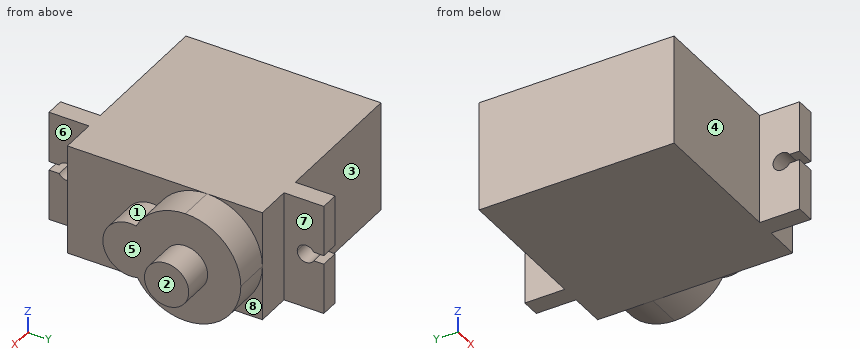
from build123d import *

# Parameters (mm, degrees)
F0_W      = 22
F0_H      = 22
F1_DEPTH  = 12.5
F3_DEPTH  = 4
F4_R      = 2.5
F5_DEPTH  = 3.5
F6_W      = 2.1
F6_H      = 12.5
F7_DEPTH  = 4.5
F9_DEPTH  = 2.1
F10_W     = 2.1
F10_H     = 12.5
F11_DEPTH = 4.5
F13_DEPTH = 2.1


with BuildPart() as f1:
    # F0 (on Top) → F1 (new body)
    with BuildSketch(Plane.XY):
        Rectangle(F0_W, F0_H)
    extrude(amount=F1_DEPTH)

    # F2 (on face) → F3 (join)
    with BuildSketch(Plane.YZ.offset(11)):
        with BuildLine():
            ThreePointArc((-0.6636140703, 3.1266552068), (1.6241725062, 0.8378190645), (4.75, 0))
            ThreePointArc((4.75, 0), (9.1694173824, 1.8305826176), (11, 6.25))
            ThreePointArc((11, 6.25), (9.1694173824, 10.6694173824), (4.75, 12.5))
            ThreePointArc((4.75, 12.5), (1.4810489541, 11.5769558905), (-0.8223385695, 9.0804668991))
            ThreePointArc((-0.8223385695, 9.0804668991), (0.9015416929, 8.0022024538), (1.5744178172, 6.0834385042))
            ThreePointArc((1.5744178172, 6.0834385042), (0.9518242766, 4.2292975847), (-0.6636140703, 3.1266552068))
        make_face()
        with BuildLine():
            ThreePointArc((-0.8223385695, 9.0804668991), (-4.568887039, 6.001564921), (-0.6636140703, 3.1266552068))
            ThreePointArc((-0.6636140703, 3.1266552068), (-1.4977801872, 6.0834385042), (-0.8223385695, 9.0804668991))
        make_face()
        with BuildLine():
            ThreePointArc((-0.8223385695, 9.0804668991), (-1.4977801872, 6.0834385042), (-0.6636140703, 3.1266552068))
            ThreePointArc((-0.6636140703, 3.1266552068), (0.9518242766, 4.2292975847), (1.5744178172, 6.0834385042))
            ThreePointArc((1.5744178172, 6.0834385042), (0.9015416929, 8.0022024538), (-0.8223385695, 9.0804668991))
        make_face()
    extrude(amount=F3_DEPTH)

    # F4 (on face) → F5 (join)
    with BuildSketch(Plane.YZ.offset(15)):
        with Locations((4.75, 6.25)):
            Circle(F4_R)
    extrude(amount=F5_DEPTH)

    # F6 (on face) → F7 (join)
    with BuildSketch(Plane.XZ.offset(11)):
        with Locations((5.95, 6.25)):
            Rectangle(F6_W, F6_H)
    extrude(amount=F7_DEPTH)

    # F8 (on face) → F9 (cut)
    with BuildSketch(Plane(origin=(4.9, 0, 0), x_dir=(0, -1, 0), z_dir=(-1, 0, 0))):
        with BuildLine():
            ThreePointArc((14.3660254038, 6.75), (14.4659258263, 6.5088190451), (14.5, 6.25))
            ThreePointArc((14.5, 6.25), (14.4659258263, 5.9911809549), (14.3660254038, 5.75))
            Line((14.3660254038, 5.75), (15.5, 5.75))
            Line((15.5, 5.75), (15.5, 6.75))
            Line((15.5, 6.75), (14.3660254038, 6.75))
        make_face()
        with BuildLine():
            ThreePointArc((14.3660254038, 5.75), (14.4659258263, 5.9911809549), (14.5, 6.25))
            ThreePointArc((14.5, 6.25), (14.4659258263, 6.5088190451), (14.3660254038, 6.75))
            ThreePointArc((14.3660254038, 6.75), (12.5, 6.25), (14.3660254038, 5.75))
        make_face()
    extrude(amount=-F9_DEPTH, mode=Mode.SUBTRACT)

    # F10 (on face) → F11 (join)
    with BuildSketch(Plane(origin=(0, 11, 0), x_dir=(-1, 0, 0), z_dir=(0, 1, 0))):
        with Locations((-5.95, 6.25)):
            Rectangle(F10_W, F10_H)
    extrude(amount=F11_DEPTH)

    # F12 (on face) → F13 (cut)
    with BuildSketch(Plane(origin=(4.9, 0, 0), x_dir=(0, -1, 0), z_dir=(-1, 0, 0))):
        with BuildLine():
            ThreePointArc((-14.3660254038, 5.75), (-13.2411809549, 5.2840741737), (-12.5, 6.25))
            ThreePointArc((-12.5, 6.25), (-13.2411809549, 7.2159258263), (-14.3660254038, 6.75))
            ThreePointArc((-14.3660254038, 6.75), (-14.5, 6.25), (-14.3660254038, 5.75))
        make_face()
        with BuildLine():
            ThreePointArc((-14.3660254038, 5.75), (-14.5, 6.25), (-14.3660254038, 6.75))
            Line((-14.3660254038, 6.75), (-15.5, 6.75))
            Line((-15.5, 6.75), (-15.5, 5.75))
            Line((-15.5, 5.75), (-14.3660254038, 5.75))
        make_face()
    extrude(amount=-F13_DEPTH, mode=Mode.SUBTRACT)


solid = f1.part
Design review of the part built by this model. Coordinates are the model's own, in mm. Face numbers are marked on the shaded views. A direction names the side the tool comes from. Round coordinates to 2 decimals unless told otherwise and drop trailing zeros. Loops run counter-clockwise (first coordinate to the right, second up) from the corner with the lowest first, then second, coordinate; pieces in that order, holes last. Notation, with made-up numbers: (13, 80) -> (52, 80) arc R28 ccw to (52, 99) -> close; hole circle Ø8 at (-3.5, -35). An arc over 180 degrees is marked (long way). Use one line per item in the form item = value. Start each with the question number.
Q1. We need section A-A on y = -13.5. Give the boundary of the cut face in (x, z), then the cut area to 4 significant figures.
Q2. For pin 1 Ø5 at (y, z) = (-14, 6.5) entering from +X; pin 2 Ø2 at (y, z) = (-13.5, 9.5) entering from -X; pin 3 Ø1 at (x, z) = (0, 7) entering from +Y; pin 4 Ø5 at (x, z) = (4, 9.5) entering from +Y, all flat-tipped, find the tip position at first contact; note any pin that passes through.
Q3. We need section B-B on y = 4. Give the boundary of the cut face in (x, z), then the cut area to 3 significant figures.
Q4. Machinability: for the marked faces 5, 6, 7 and 8, which of the approach directions +Z, -Z, +X, -X, +Y, -Y give a long, thin tool a straight path to every point of the face, cutting with its end or side? Answer none if there is none.
Q5. We need section C-C on x = 1.75. Give the boundary of the cut face in (y, z).
Q6. Draft analysis for pull direction Y (two halves, no side actions). For the marked faces 1, 2, 3 and 4, state which applies: +Y half, -Y half, draft (parallel to the pull), parting line (faces both ways), or undercut.
Q7. Wall thickness on line 1 along Z through (x, y) = (6.35, -13.5); line 2 along X through (y, z) = (13, 9.75); line 3 along Y through (x, z) = (-7.5, 6.25): over which ranges is each line inside the solid? List them lowest first. Write a range as [from, to].
Calculated:
q1.outline = (4.9, 0) -> (7, 0) -> (7, 5.25) -> (4.9, 5.25) -> close; (4.9, 7.25) -> (7, 7.25) -> (7, 12.5) -> (4.9, 12.5) -> close
q1.area = 22.05 mm²
q2.pin_1 = 7
q2.pin_2 = 4.9
q2.pin_3 = 11
q2.pin_4 = 15.5
q3.outline = (-11, 0) -> (11, 0) -> (11, 0.05) -> (15, 0.05) -> (15, 3.87) -> (18.5, 3.87) -> (18.5, 8.63) -> (15, 8.63) -> (15, 12.45) -> (11, 12.45) -> (11, 12.5) -> (-11, 12.5) -> close
q3.area = 341 mm²
q4.face_5 = +X
q4.face_6 = +Z, -Z, +X, -Y
q4.face_7 = +Z, -Z, +X, +Y
q4.face_8 = -Z, +X, +Y
q5.outline = (-11, 0) -> (11, 0) -> (11, 12.5) -> (-11, 12.5) -> close
q6.face_1 = undercut
q6.face_2 = draft
q6.face_3 = +Y half
q6.face_4 = -Y half
q7.line_1 = [0, 5.25], [7.25, 12.5]
q7.line_2 = [4.9, 7]
q7.line_3 = [-11, 11]
